from build123d import *

# Parameters (mm, degrees)
F0_W     = 95.25
F0_H     = 63.5
F1_DEPTH = 50.8
F3_DEPTH = 63.501
F5_DEPTH = 25.4
F6_R     = 9.525
F7_DEPTH = 25.4


with BuildPart() as f1:
    # F0 (on Top) → F1 (new body)
    with BuildSketch(Plane.XY):
        with Locations((-29.448411174, -18.1773232762)):
            Rectangle(F0_W, F0_H)
    extrude(amount=F1_DEPTH)

    # F2 (on face) → F3 (cut, through all)
    with BuildSketch(Plane.XZ.offset(49.9273232762)):
        with BuildLine():
            Line((-77.073411174, 50.8), (-77.073411174, 0))
            Line((-77.073411174, 0), (-39.1752533615, 23.0941344053))
            Line((-39.1752533615, 23.0941344053), (-18.6140239239, 23.0941344053))
            ThreePointArc((-18.6140239239, 23.0941344053), (-1.3716503463, 42.6423735776), (18.176588826, 25.4))
            Line((18.176588826, 25.4), (18.176588826, 50.8))
            Line((18.176588826, 50.8), (-77.073411174, 50.8))
        make_face()
    extrude(amount=-F3_DEPTH, mode=Mode.SUBTRACT)

    # F4 (on face) → F5 (cut)
    with BuildSketch(Plane.YZ.offset(18.176588826)):
        with BuildLine():
            ThreePointArc((-24.7437144876, 12.7), (-34.2687144876, 22.225), (-43.7937144876, 12.7))
            Line((-43.7937144876, 12.7), (-24.7437144876, 12.7))
        make_face()
        with BuildLine():
            Line((-24.7437144876, 12.7), (-43.7937144876, 12.7))
            ThreePointArc((-43.7937144876, 12.7), (-34.2687144876, 3.175), (-24.7437144876, 12.7))
        make_face()
        with BuildLine():
            ThreePointArc((-43.7937144876, 12.7), (-34.2687144876, 3.175), (-24.7437144876, 12.7))
            Line((-24.7437144876, 12.7), (-43.7937144876, 12.7))
        make_face()
    extrude(amount=-F5_DEPTH, mode=Mode.SUBTRACT)

    # F6 (on face) → F7 (cut)
    with BuildSketch(Plane.YZ.offset(18.176588826)):
        with Locations((0, 12.7)):
            Circle(F6_R)
    extrude(amount=-F7_DEPTH, mode=Mode.SUBTRACT)


solid = f1.part
Can you work these out from the model? Positions are in its coordinate system, mm. A direction names the side the tool comes from. Coordinates: 2 decimals unless noted, no trailing zeros. Loops run counter-clockwise (first coordinate to the right, second up) from the corner with the lowest first, then second, coordinate; pieces in that order, holes last. Notation, with made-up numbers: M -18.5,9.25 L 19.5,9.25 A26 ccw 19.5,38.25 Z; hole C 80,-25 d10. An arc over 180 degrees is marked long. Answer as CSV lines item,"result". Start each with the question number.
1. Suppose I cut it at B-B, the plane x = 7. List the corners of the cut face in (y, z) for me (3 decimals).
2. Suppose I cut it at C-C, the plane z = 12.7. List the corners of the cut face in (x, y) for me (3 decimals), plus the area to 3 significant figures.
3. If I drill on probe 1 along Y at (x, z) = (10, 12); probe 2 along Z at (x, y) = (13.5, 7); probe 3 along Z at (x, y) = (-20, -22), over which ranges is the centre line in solid material (lowest first)? Write a range as [from, to].
4. Suppose I cut it at D-D, the plane x = -36.5. List the corners of the cut face in (y, z) for me.
5. Thinking about a two-plate mould opening in Z: for faces 4 (the face through (5.65, -36.33, 3.4)), 5 (the face through (-58.39, -18.622, 11.385)), 6 (the face through (-20, 13.573, 16)), 7 (the face through (-30, -18, 0)), which applies, +Z half, -Z half, draft (parallel to the pull), parting line (faces both ways), or undercut?
6. For faces 1 (the face through (-29, -19, 23.094)), 2 (the face through (-7.223, 0, 13)), 3 (the face through (-20, -49.927, 16)), which set-ups out of +Z, -Z, +X, -X, +Y, -Y let a thin tool reach every point of the face, with its end or its side?
7. Suppose I cut it at A-A, the plane y = -12. List the corners of the cut face in (x, z) for me, plus the area to 3 significant figures.
8. For pin 1 Ø6 at (x, y) = (-52, -42.5) entering from +Z; pin 2 Ø9.5 at (y, z) = (-31.5, 9) entering from +X; pin 3 Ø4 at (x, y) = (-43.5, -14.5) entering from -Z; pin 4 Ø22.5 at (x, y) = (-28, -28.5) entering from +Z, each with a flat end and sliding along its axis, tell me the tip position at first contact or that it passes through.
Output:
1,outline,"M -49.927,0 L 13.573,0 L 13.573,41.206 L -49.927,41.206 Z; hole C -34.269,12.7 d19.05; hole C 0,12.7 d19.05"
2,outline,"M -56.232,-49.927 L 18.177,-49.927 L 18.177,-43.794 L -7.223,-43.794 L -7.223,-24.744 L 18.177,-24.744 L 18.177,-9.525 L -7.223,-9.525 L -7.223,9.525 L 18.177,9.525 L 18.177,13.573 L -56.232,13.573 Z"
2,area,"3,760 mm^2"
3,probe 1,"y = [-49.93, -43.77], [-24.77, -9.5], [9.5, 13.57]"
3,probe 2,"z = [0, 6.24], [19.16, 36.56]"
3,probe 3,"z = [0, 23.09]"
4,outline,"M -49.93,0 L 13.57,0 L 13.57,23.09 L -49.93,23.09 Z"
5,face 4,"undercut"
5,face 5,"+Z half"
5,face 6,"draft"
5,face 7,"-Z half"
6,face 1,"+Z, -X, +Y, -Y"
6,face 2,"+X"
6,face 3,"+Z, -Z, +X, -X, -Y"
7,outline,"M -77.07,0 L 18.18,0 L 18.18,25.4 A18.43 ccw -18.61,23.09 L -39.18,23.09 Z"
7,area,"2,340 mm^2"
8,pin 1,"stops at z = 17.11"
8,pin 2,"stops at x = -7.22"
8,pin 3,"stops at z = 0"
8,pin 4,"stops at z = 32.4"
